Autodesk Inventor part; units mm, degrees
ref_plane "YZ Plane" through (0, 0, 0) normal (1, 0, 0) x (0, 1, 0)
ref_plane "XZ Plane" through (0, 0, 0) normal (0, 1, 0) x (-1, 0, 0)
ref_plane "XY Plane" through (0, 0, 0) normal (0, 0, 1) x (1, 0, 0)
ref_plane "Work Plane1" through (-244.5168, 0, -292.1078) normal (0, -1, 0) x (1, 0, 0)
sketch "Sketch1" plane through (-244.5168, 0, -292.1078) normal (0, -1, 0) x (1, 0, 0)
  line L0 (-82.2349, -443.0164) -> (-82.2349, 4.1434)
  line L1 (16.0565, -523.4999) -> (-89.6349, -493.4083)
  line L2 (-82.2349, 4.1434) -> (116.5991, 288.1078)
  line L3 (116.5991, 288.1078) -> (240.5168, 288.1078)
  line L4 (590.8332, -25.4546) -> (443.4975, 290.5078)
  line L5 (590.8332, -523.4999) -> (590.8332, -25.4546)
  point P0 (244.5168, 292.1078)
sketch "Sketch2" plane through (-244.5168, 0, -292.1078) normal (0, -1, 0) x (1, 0, 0)
  line L0 (16.0565, -523.4999) -> (-82.2349, -495.4665)
  line L1 (-82.2349, -495.4665) -> (-82.2349, 4.1434)
  line L2 (-82.2349, 4.1434) -> (116.5991, 288.1078)
  line L3 (116.5991, 288.1078) -> (443.4975, 290.5078)
  line L4 (443.4975, 290.5078) -> (590.8332, -25.4546)
  line L5 (590.8332, -25.4546) -> (590.8332, -523.4999)
  line L6 (590.8332, -523.4999) -> (16.0565, -523.4999)
  point P0 (244.5168, 292.1078)
extrude "Plate extrude" add sketch "Sketch2" against normal blind 1.6
sketch "Sketch3" plane through (-244.5168, 0, -292.1078) normal (0, -1, 0) x (1, 0, 0)
  circle A0 centre (303.4237, -47.9675) radius 80.5 construction
  circle A1 centre (303.4237, -47.7578) radius 75 construction
  line L0 (153.4237, 102.2422) -> (453.4237, 102.2422)
  line L1 (453.4237, 102.2422) -> (453.4237, -197.7578)
  line L2 (453.4237, -197.7578) -> (153.4237, -197.7578)
  line L3 (153.4237, -197.7578) -> (153.4237, 102.2422)
  line L4 (153.4237, 102.2422) -> (453.4237, -197.7578) construction
  line L5 (453.4237, 102.2422) -> (153.4237, -197.7578) construction
  point P0 (244.5168, 292.1078)
  dimension "d3" = 300
  dimension "d4" = 300
extrude "Tailstock door" [suppressed]
sketch "Sketch4" plane through (-244.5168, 0, -292.1078) normal (0, -1, 0) x (1, 0, 0)
  circle A0 centre (303.4237, -47.7578) radius 75 construction
  circle A1 centre (303.4237, -47.7578) radius 81.28
  circle A2 centre (303.4237, -47.9675) radius 80.5 construction
  point P0 (244.5168, 292.1078)
  dimension "d7" = 162.56
  dimension "d8" = 161
extrude "Headstock cut out" [suppressed]
sketch "Sketch5" plane through (-244.5168, 1.6, -292.1078) normal (0, 1, 0) x (1, 0, 0)
  point P0 (244.5168, -292.1078)
  point P1 (303.4237, 47.9675)
properties part number "side cover plate Base"
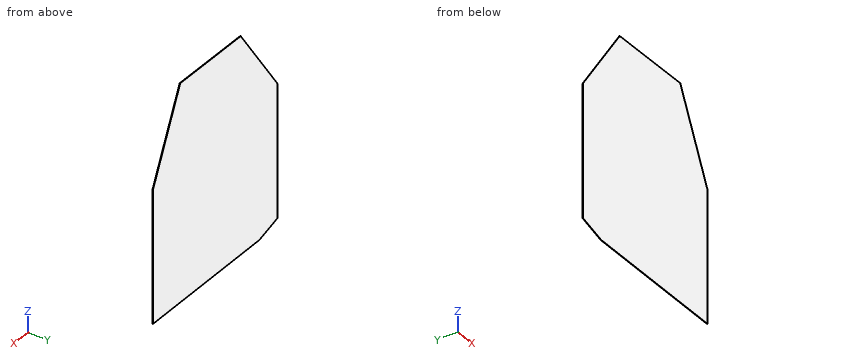
The listing builds one solid part. Answer for the finished solid, in the listing's coordinates (mm). Give positions to 0.01 mm unless a question says otherwise; leave off trailing zeros. Loops run counter-clockwise (first coordinate to the right, second up) from the corner with the lowest first, then second, coordinate; pieces in that order, holes last. Notation, with made-up numbers: (-2, 38) - (4, 38) arc R16 cw to (4, 65) - close; hole circle Ø3 at (-6.75, 50.5). An arc over 180 degrees is marked (long way). Write each question's results on one line, items separated by ' | '.
1. Consider probe 1 along Z at (x, y) = (-63, 0.6); probe 2 along Z at (x, y) = (-122.5, 0.2); probe 3 along X at (y, z) = (0.95, -156.5). Determine where each line is inside the solid, lowest interval first. Write a range as from..to.
Resolved:
probe 1: z = -815.61..-3.52 | probe 2: z = -815.61..-3.96 | probe 3: x = -234.7..271.21
2. Find section A-A, the plane y = 1.2. Write down the section's boundary in (x, z), then the cut area to 3 significant figures.
Resolved:
outline: (-326.75, -787.57) - (-228.46, -815.61) - (346.32, -815.61) - (346.32, -317.56) - (198.98, -1.6) - (-127.92, -4) - (-326.75, -287.96) - close | area: 494,000 mm^2
3. Find section B-B, the plane z = -238. Write down the section's boundary in (x, y), then the cut area to 3 significant figures.
Resolved:
outline: (-291.77, 0) - (309.22, 0) - (309.22, 1.6) - (-291.77, 1.6) - close | area: 962 mm^2
4. Find section C-C, the plane x = -177.5. Write down the section's boundary in (y, z), then the cut area to 3 significant figures.
Resolved:
outline: (0, -815.61) - (1.6, -815.61) - (1.6, -74.81) - (0, -74.81) - close | area: 1,190 mm^2
